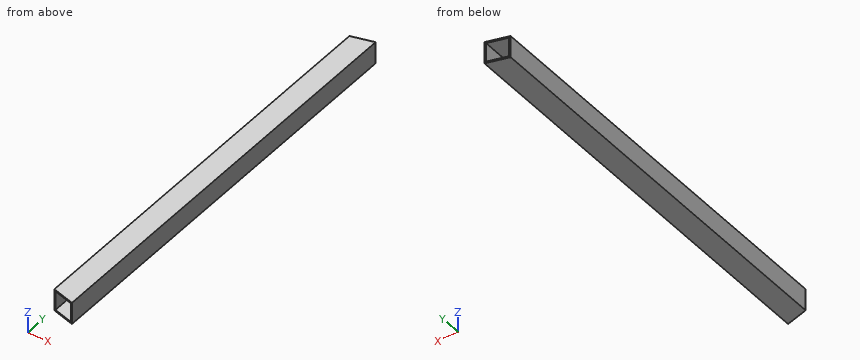
from build123d import *

# Parameters (mm, degrees)
F0_W     = 25.4
F0_H     = 25.4
F0_W_2   = 22.225
F0_H_2   = 22.225
F1_DEPTH = 242.57
F3_DEPTH = 25.401


# Not quite as in the source:
# - a pattern or mirror of a feature is missing from the dataset's text; its kind, count and spacing are read off the source's solid


with BuildPart() as f1:
    # F0 (on Front) → F1 (new body, symmetric)
    with BuildSketch(Plane.XZ):
        Rectangle(F0_W, F0_H)
        Rectangle(F0_W_2, F0_H_2, mode=Mode.SUBTRACT)
    extrude(amount=F1_DEPTH, both=True)

    # F2 (on face) → F3 (cut, through all)
    with BuildSketch(Plane.XY.offset(12.7)):
        Polygon((12.7, 242.57), (-12.7, 242.57), (-12.7, 235.6213463057), align=None)
    f3 = extrude(amount=-F3_DEPTH, mode=Mode.SUBTRACT)

    # F3_copies: F3 across plane
    add(f3.mirror(Plane(origin=(0, 0, 0), x_dir=(0, 0, -1), z_dir=(0, -1, 0))), mode=Mode.SUBTRACT)


solid = f1.part
Geometry: final body of the model. Coordinates: model frame, mm. Round coordinates to 2 decimals unless told otherwise and drop trailing zeros. Loops run counter-clockwise (first coordinate to the right, second up) from the corner with the lowest first, then second, coordinate; pieces in that order, holes last. Notation, with made-up numbers: M -38,64.25 L -23,64.25 A22 cw -23,70.25 Z; hole C -5.75,-34.75 d11. An arc over 180 degrees is marked long. One line per question, with ' | ' between items.
(1) Material intervals for line 1 along X through (y, z) = (-160, 8), sorted ascending. Write a range as from..to.
Check result:
line 1: x = -12.7..-11.11, 11.11..12.7
(2) Cut plane A-A on y = 61. Return the cut outline in (x, z), plus the area to 3 significant figures.
Check result:
outline: M -12.7,-12.7 L 12.7,-12.7 L 12.7,12.7 L -12.7,12.7 Z; hole M -11.11,-11.11 L 11.11,-11.11 L 11.11,11.11 L -11.11,11.11 Z | area: 151 mm2
(3) Cut plane C-C on x = -6. Return the cut outline in (y, z), plus the area to 3 significant figures.
Check result:
outline: M -237.45,-12.7 L 237.45,-12.7 L 237.45,-11.11 L -237.45,-11.11 Z; M -237.45,11.11 L 237.45,11.11 L 237.45,12.7 L -237.45,12.7 Z | area: 1,510 mm2
(4) Contact query for a flat-ended pin moving along its axis: P1, Ø5, axis at x = 3.5, z = -6.5, coming from the -Y side. Output: stop coordinate, or through.
Check result:
P1: passes through
(5) Cut plane B-B on z = 1. Return the cut outline in (x, y).
Check result:
outline: M -12.7,-235.62 L -11.11,-236.06 L -11.11,236.06 L -12.7,235.62 Z; M 11.11,-242.14 L 12.7,-242.57 L 12.7,242.57 L 11.11,242.14 Z
